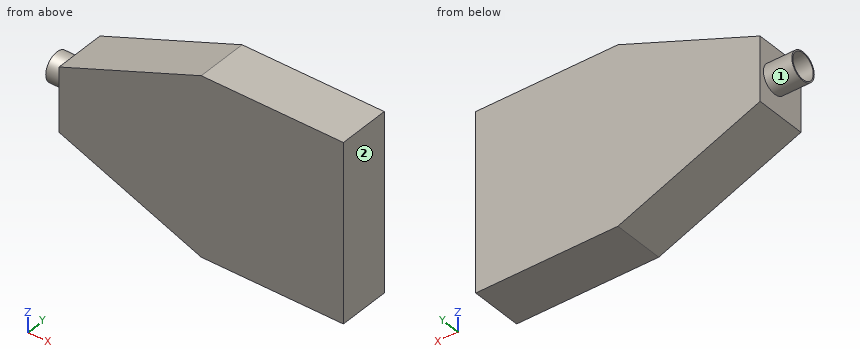
from build123d import *

# Parameters (mm, degrees)
SKETCH1_W           = 100
SKETCH1_H           = 125
BOSS_EXTRUDE1_DEPTH = 36.5
SKETCH27_R          = 10
BOSS_EXTRUDE2_DEPTH = 20
SKETCH28_R          = 9.1
CUT_EXTRUDE11_DEPTH = 20


with BuildPart() as part:
    # Sketch1 → Boss-Extrude1 (new body)
    with BuildSketch(Plane(origin=(0, 0, 0), x_dir=(1, 0, 0), z_dir=(0, 1, 0))):
        Polygon((-150, 22.5), (-150, -22.5), (-50, -62.5), (-50, 62.5), align=None)
        Rectangle(SKETCH1_W, SKETCH1_H)
    extrude(amount=BOSS_EXTRUDE1_DEPTH)

    # Sketch27 → Boss-Extrude2 (add)
    with BuildSketch(Plane.ZY.offset(150)):
        with Locations((0, 23.5)):
            Circle(SKETCH27_R)
    extrude(amount=BOSS_EXTRUDE2_DEPTH)

    # Sketch28 → Cut-Extrude11 (cut)
    with BuildSketch(Plane.ZY.offset(170)):
        with Locations((0, 23.5)):
            Circle(SKETCH28_R)
    extrude(amount=-CUT_EXTRUDE11_DEPTH, mode=Mode.SUBTRACT)


solid = part.part
Input: part model. Units: mm. Frame: model coordinates. Face numbers are marked on the shaded views. A direction names the side the tool comes from. Coordinates: 2 decimals unless noted, no trailing zeros. Loops run counter-clockwise (first coordinate to the right, second up) from the corner with the lowest first, then second, coordinate; pieces in that order, holes last.
Q1. Set-up query: the marked faces 1 and 2. Return all of +Z, -Z, +X, -X, +Y, -Y with unobstructed straight access to the full face (end or side cutting, diameter ignored); none if empty.
Q2. Cut plane A-A (z = 0). Output: boundary loops of the cut face in (x, y), then the cut area to 3 significant figures.
Q3. Cut plane B-B (x = -67.5). Output: boundary loops of the cut face in (y, z).
Q4. Material intervals for line 1 (Y direction, x = -154.25, z = 0); line 2 (X direction, y = 19.5, z = 6); line 3 (Z direction, x = -143, y = 5), sorted ascending.
Q5. Cut plane D-D (z = -38). Output: boundary loops of the cut face in (x, y).
Q6. Contact query for flat-ended pins moving along their axis: pin 1 (14.5 mm diameter, centred on y = 23.5, z = 0, fed in from -X); pin 2 (1.5 mm diameter, centred on x = -52.5, y = 16.5, fed in from -Z); pin 3 (12 mm diameter, centred on x = -125.5, y = 23.5, fed in from -Z). Output: stop coordinate, or through.
Q7. Cut plane C-C (y = 18.5). Output: boundary loops of the cut face in (x, z), then the cut area to 3 significant figures.
Working result:
1. face 1: -X
1. face 2: +Z, -Z, +X, +Y, -Y
2. outline: (-170, 13.5) - (-150, 13.5) - (-150, 0) - (50, 0) - (50, 36.5) - (-150, 36.5) - (-150, 33.5) - (-170, 33.5) - (-170, 32.6) - (-150, 32.6) - (-150, 14.4) - (-170, 14.4) - close
2. area: 7,340 mm2
3. outline: (0, -55.5) - (36.5, -55.5) - (36.5, 55.5) - (0, 55.5) - close
4. line 1: y = 13.5 to 14.4, 32.6 to 33.5
4. line 2: x = -150 to 50
4. line 3: z = -25.3 to 25.3
5. outline: (-111.25, 0) - (50, 0) - (50, 36.5) - (-111.25, 36.5) - close
6. pin 1: stops at x = -150
6. pin 2: stops at z = -61.8
6. pin 3: stops at z = -34.7
7. outline: (-170, -8.66) - (-150, -8.66) - (-150, -22.5) - (-50, -62.5) - (50, -62.5) - (50, 62.5) - (-50, 62.5) - (-150, 22.5) - (-150, 8.66) - (-170, 8.66) - (-170, 7.6) - (-150, 7.6) - (-150, -7.6) - (-170, -7.6) - close
7. area: 21,000 mm2
